Build history of the part. All positions in model axes, mm. Face numbers are marked on the shaded views. A direction names the side the tool comes from. Coordinates: 2 decimals unless noted, no trailing zeros. Order: outer loops, then holes, each group sorted by start corner. A loop starts at its lowest first (then second) coordinate and runs counter-clockwise, first axis right, second up. Notation, with made-up numbers: (49, -5) - (63, -5) arc R20 cw to (63, 17) - close; hole circle Ø8 at (74.25, -4.5). An arc over 180 degrees is marked (long way). Write each question's results on one line, items separated by ' | '.
from build123d import *

# Parameters (mm, degrees)
EXTRUDE_1_DEPTH      = 90
EXTRUDE_1_DEPTH_BACK = 90
SKETCH_1_R           = 32
SKETCH_2_W           = 74
SKETCH_2_H           = 58
EXTRUDE_2_DEPTH      = 300
SKETCH_3_W           = 4
SKETCH_3_H           = 40
EXTRUDE_3_DEPTH      = 300
EXTRUDE_4_DEPTH      = 55
EXTRUDE_4_DEPTH_BACK = 55
SKETCH_4_R           = 53
SKETCH_4_R_2         = 35


with BuildPart() as part:
    # Sketch 1 → Extrude 1 (new, two sides: drawn at the far end of the back side and taken through both)
    with BuildSketch(Plane(origin=(0, 0, 0), x_dir=(1, 0, 0), z_dir=(0, 1, 0)).offset(-EXTRUDE_1_DEPTH_BACK)):
        with Locations(Location((0, 0, 0), (0, 0, 270))):
            Circle(SKETCH_1_R)
    extrude(amount=EXTRUDE_1_DEPTH + EXTRUDE_1_DEPTH_BACK)

    # Sketch 2 → Extrude 2 (add)
    with BuildSketch(Plane.XY):
        Rectangle(SKETCH_2_W, SKETCH_2_H)
    extrude(amount=EXTRUDE_2_DEPTH)

    # Sketch 3 → Extrude 3 (add)
    with BuildSketch(Plane.XY):
        with Locations((39, 0)):
            Rectangle(SKETCH_3_W, SKETCH_3_H)
        with Locations((-39, 0)):
            Rectangle(SKETCH_3_W, SKETCH_3_H)
    extrude(amount=EXTRUDE_3_DEPTH)

    # Sketch 4 → Extrude 4 (add, two sides: drawn at the far end of the back side and taken through both)
    with BuildSketch(Plane(origin=(0, 0, 0), x_dir=(1, 0, 0), z_dir=(0, 1, 0)).offset(-EXTRUDE_4_DEPTH_BACK)):
        with Locations(Location((0, -300, 0), (0, 0, 270))):
            Circle(SKETCH_4_R)
        with Locations(Location((0, -300, 0), (0, 0, 270))):
            Circle(SKETCH_4_R_2, mode=Mode.SUBTRACT)
    extrude(amount=EXTRUDE_4_DEPTH + EXTRUDE_4_DEPTH_BACK)


solid = part.part
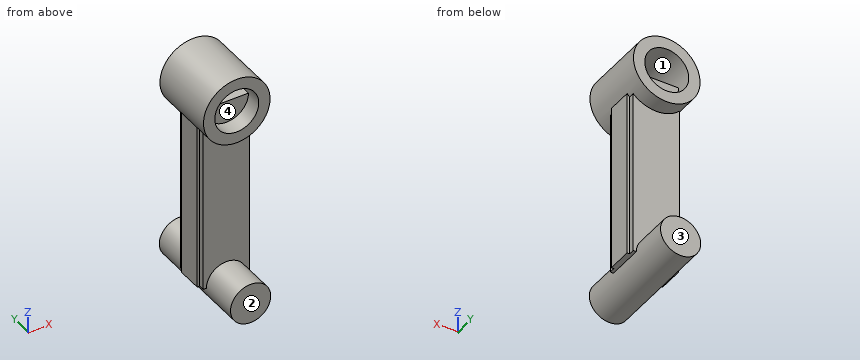
1. Tool access for the marked faces 1 and 2: list every direction of +Z, -Z, +X, -X, +Y, -Y with a clear straight run to the whole face (end or side of a thin tool).
Solved:
face 1: none | face 2: +Z, -Z, +X, -X, -Y
2. Band-saw the part on D-D on y = -39.5. Give the cut face in (x, z).
Solved:
outline: circle Ø106 at (0, 300); circle Ø64 at (0, 0); hole circle Ø70 at (0, 300)
3. Band-saw the part on A-A on y = 8.5. Give the cut face in (x, z).
Solved:
outline: (-41, 0) - (-32, 0) arc R32 ccw to (32, 0) - (41, 0) - (41, 266.41) arc R53 ccw (long way) to (-41, 266.41) - close; hole (-35, 300) - (35, 300) arc R35 ccw to start
4. Probe line 1 (Z direction, x = 2, y = -41.5); line 2 (Z direction, x = -7, y = 32); line 3 (Z direction, x = 4, y = -6.5). List the from-to ranges inside material, lowest first.
Solved:
line 1: z = -31.94 to 31.94, 247.04 to 265.06, 334.94 to 352.96 | line 2: z = -31.22 to 31.22, 247.46 to 265.71, 334.29 to 352.54 | line 3: z = -31.75 to 300, 334.77 to 352.85
5. Band-saw the part on C-C on z = 328. Give the cut face in (x, y), then the cut area to 3 significant figures.
Solved:
outline: (-45, -55) - (-21, -55) - (-21, 55) - (-45, 55) - close; (21, -55) - (45, -55) - (45, 55) - (21, 55) - close | area: 5,280 mm2
6. Band-saw the part on B-B on x = 0. Give the cut face in (y, z), then the cut area to 3 significant figures.
Solved:
outline: (-90, -32) - (90, -32) - (90, 32) - (29, 32) - (29, 247) - (55, 247) - (55, 265) - (29, 265) - (29, 300) - (-29, 300) - (-29, 265) - (-55, 265) - (-55, 247) - (-29, 247) - (-29, 32) - (-90, 32) - close; (-55, 335) - (55, 335) - (55, 353) - (-55, 353) - close | area: 30,000 mm2
7. Drop flat-ended pins along their axis: pin 1 Ø3 at (x, z) = (-39.5, 105) entering from +Y; pin 2 Ø6 at (y, z) = (2.5, 105.5) entering from -X; pin 3 Ø10.5 at (x, z) = (-14.5, 286) entering from +Y. Give the stop position or say it passes through.
Solved:
pin 1: stops at y = 20 | pin 2: stops at x = -41 | pin 3: stops at y = 29
8. Two-plate mould, pull along Z, no slides. Class the marked faces 3 and 4: +Z half, -Z half, draft (parallel to the pull), parting line (faces both ways), or undercut.
Solved:
face 3: draft | face 4: undercut
